```python
from build123d import *

# Parameters (mm, degrees)
PAD001_DEPTH          = 37.5
SKETCH_R              = 80
SKETCH_R_2            = 20
PAD_DEPTH             = 45
SKETCH001_R           = 30
POCKET_DEPTH          = 16
POCKET001_DEPTH       = 20
POLARPATTERN_COUNT    = 4
SKETCH003_R           = 9
POCKET002_DEPTH       = 486.41188
POLARPATTERN001_COUNT = 4


with BuildPart() as pad001:
    # Sketch004 → Pad001 (new body, symmetric)
    with BuildSketch(Plane.YZ):
        Polygon((0, 45), (-85, 33.054029), (-85, 45), align=None)
    extrude(amount=PAD001_DEPTH, both=True)


with BuildPart() as part_mirroring:
    # Part__Mirroring: instance of Pad001
    add(pad001.part.mirror(Plane(origin=(0, 0, 0), x_dir=(1, 0, 0), z_dir=(0, 1, 0))))


with BuildPart() as cut001:
    # Sketch → Pad (new body)
    with BuildSketch(Plane.XY):
        Circle(SKETCH_R)
        Circle(SKETCH_R_2, mode=Mode.SUBTRACT)
    extrude(amount=PAD_DEPTH)

    # Sketch001 → Pocket (cut)
    with BuildSketch(Plane.XY.offset(45)):
        Circle(SKETCH001_R)
    extrude(amount=-POCKET_DEPTH, mode=Mode.SUBTRACT)

    # Sketch002 → Pocket001 (cut)
    with BuildSketch(Plane.XY.offset(45)):
        with BuildLine():
            ThreePointArc((-18, -77.948701), (0, -80), (18, -77.948701))
            Line((18, -77.948701), (18, -62))
            ThreePointArc((18, -62), (-2.4e-05, -44), (-18, -62.000049))
            Line((-18, -77.948701), (-18, -62.000049))
        make_face()
    pocket001 = extrude(amount=-POCKET001_DEPTH, mode=Mode.SUBTRACT)

    # PolarPattern: Pocket001 ×4 about axis
    polarpattern_axis = Axis((0, 0, 45), (0, 0, 1))
    for i in range(1, POLARPATTERN_COUNT):
        add(pocket001.rotate(polarpattern_axis, i * 360 / POLARPATTERN_COUNT), mode=Mode.SUBTRACT)

    # Sketch003 → Pocket002 (cut, through all)
    with BuildSketch(Plane.XY.offset(25)):
        with Locations((0, -62)):
            Circle(SKETCH003_R)
    pocket002 = extrude(amount=-POCKET002_DEPTH, mode=Mode.SUBTRACT)

    # PolarPattern001: Pocket002 ×4 about axis
    polarpattern001_axis = Axis((0, 0, 25), (0, 0, 1))
    for i in range(1, POLARPATTERN001_COUNT):
        add(pocket002.rotate(polarpattern001_axis, i * 360 / POLARPATTERN001_COUNT), mode=Mode.SUBTRACT)

    # Cut: cut Part__Mirroring
    add(part_mirroring.part, mode=Mode.SUBTRACT)

    # Cut001: cut Pad001
    add(pad001.part, mode=Mode.SUBTRACT)


solid = cut001.part
```
Geometry: final body of the model. Coordinates: model frame, mm. A direction names the side the tool comes from. Coordinates: 2 decimals unless noted, no trailing zeros. Order: outer loops, then holes, each group sorted by start corner. A loop starts at its lowest first (then second) coordinate and runs counter-clockwise, first axis right, second up.
Item 1: Draft query along Y for faces 6 (the face through (0, -44, 32)), 7 (the face through (70.786, -1.951, 12.675)), 8 (the face through (0.52, 38.43, 39.6)), 9 (the face through (70, -18, 35)). Return one class per face: released by +Y, released by -Y, zero draft, split by the parting line, or undercut.
Answer:
face 6: released by -Y
face 7: undercut
face 8: released by +Y
face 9: undercut
Item 2: Access query for faces 1 (the face through (37.5, -51, 42)), 2 (the face through (0, 44, 32)), 3 (the face through (-29.97, 1.32, 35.33)), 4 (the face through (-74, 0, 25)), 5 (the face through (74, 0, 25)). Directions: +Z, -Z, +X, -X, +Y, -Y. A direction counts if a zero-diameter tool reaches every point of the face in a straight line with its end or side. Return the directions, or none.
Answer:
face 1: +Z, -Y
face 2: +Z, +Y
face 3: +Z
face 4: +Z, -X
face 5: +Z, +X
Item 3: Section query C-C (x = 0). Output: boundary loops of the cut face in (y, z).
Answer:
outline: (-80, 0) - (-71, 0) - (-71, 25) - (-80, 25) - close; (-53, 0) - (-20, 0) - (-20, 29) - (-30, 29) - (-30, 40.78) - (-44, 38.82) - (-44, 25) - (-53, 25) - close; (20, 0) - (53, 0) - (53, 25) - (44, 25) - (44, 38.82) - (30, 40.78) - (30, 29) - (20, 29) - close; (71, 0) - (80, 0) - (80, 25) - (71, 25) - close
Item 4: Material intervals for line 1 along Y through (x, z) = (0, 4); line 2 along Z through (x, y) = (60.5, 10); line 3 along X through (y, z) = (62, 15), sorted ascending.
Answer:
line 1: y = -80 to -71, -53 to -20, 20 to 53, 71 to 80
line 2: z = 0 to 25
line 3: x = -50.56 to -9, 9 to 50.56
Item 5: Section query D-D (y = -39). Output: boundary loops of the cut face in (x, z), then the cut area to 3 significant figures.
Answer:
outline: (-69.85, 0) - (69.85, 0) - (69.85, 45) - (37.5, 45) - (37.5, 39.52) - (-37.5, 39.52) - (-37.5, 45) - (-69.85, 45) - close
area: 5,880 mm2
Item 6: Contact query for flat-ended pins moving along their axis: P1, Ø8, axis at x = -44, z = 9, coming from the +Y side; P2, Ø2, axis at x = 28.5, y = -4, coming from the -Z side; P3, Ø3, axis at y = -26.5, z = 26.5, coming from the -X side; P4, Ø13, axis at x = -73, z = 30, coming from the +Y side. Output: stop coordinate, or through.
Answer:
P1: stops at y = 69.28
P2: stops at z = 0
P3: stops at x = -75.99
P4: stops at y = 44.47
Item 7: Section query A-A (x = -65). Output: boundary loops of the cut face in (y, z).
Answer:
outline: (-46.64, 0) - (-8.49, 0) - (-8.49, 25) - (-18, 25) - (-18, 45) - (-46.64, 45) - close; (8.49, 0) - (46.64, 0) - (46.64, 45) - (18, 45) - (18, 25) - (8.49, 25) - close
Item 8: Section query B-B (y = -57.5). Output: boundary loops of the cut face in (x, z).
Answer:
outline: (-55.62, 0) - (-7.79, 0) - (-7.79, 25) - (-17.43, 25) - (-17.43, 36.92) - (-37.5, 36.92) - (-37.5, 45) - (-55.62, 45) - close; (7.79, 0) - (55.62, 0) - (55.62, 45) - (37.5, 45) - (37.5, 36.92) - (17.43, 36.92) - (17.43, 25) - (7.79, 25) - close
